Design review of the part built by this model. Coordinates are the model's own, in mm. A direction names the side the tool comes from. Round coordinates to 2 decimals unless told otherwise and drop trailing zeros. Loops run counter-clockwise (first coordinate to the right, second up) from the corner with the lowest first, then second, coordinate; pieces in that order, holes last. Notation, with made-up numbers: (-15.75, 81.5) - (0.25, 81.5) arc R6 cw to (0.25, 85.5) - close; hole circle Ø10 at (14, 35.25). An arc over 180 degrees is marked (long way). One line per question, with ' | ' between items. Start each with the question number.
from build123d import *

# Parameters (mm, degrees)
SKETCH1_W                = 53.5
SKETCH1_H                = 68.5
BOSS_EXTRUDE1_DEPTH      = 15
BOSS_EXTRUDE2_DEPTH      = 2.5
BOSS_EXTRUDE2_DEPTH_BACK = 15
SKETCH2_W                = 57.5
SKETCH2_H                = 72.5
SKETCH2_W_2              = 53.5
SKETCH2_H_2              = 68.5
SKETCH3_W                = 2.7
SKETCH3_H                = 68.5
CUT_EXTRUDE1_DEPTH       = 1.7
SKETCH4_R                = 1.3
CUT_EXTRUDE2_DEPTH       = 7
SKETCH5_W                = 15
SKETCH5_H                = 12
SKETCH5_R                = 2.5
SKETCH5_W_2              = 12
SKETCH5_H_2              = 15
BOSS_EXTRUDE3_DEPTH      = 3.5
FILLET1_R                = 5
FILLET2_R                = 3


with BuildPart() as part:
    # Sketch1 → Boss-Extrude1 (new body)
    with BuildSketch(Plane.XY):
        with Locations((26.75, 34.25)):
            Rectangle(SKETCH1_W, SKETCH1_H)
    extrude(amount=BOSS_EXTRUDE1_DEPTH)

    # Sketch2 → Boss-Extrude2 (add, two sides: drawn at the far end of the back side and taken through both)
    with BuildSketch(Plane.XY.offset(15).offset(-BOSS_EXTRUDE2_DEPTH_BACK)):
        with Locations((26.75, 34.25)):
            Rectangle(SKETCH2_W, SKETCH2_H)
        with Locations((26.75, 34.25)):
            Rectangle(SKETCH2_W_2, SKETCH2_H_2, mode=Mode.SUBTRACT)
    extrude(amount=BOSS_EXTRUDE2_DEPTH + BOSS_EXTRUDE2_DEPTH_BACK)

    # Sketch3 → Cut-Extrude1 (cut)
    with BuildSketch(Plane.XY.offset(15)):
        with Locations((1.85, 34.25)):
            Rectangle(SKETCH3_W, SKETCH3_H)
        with Locations((51.65, 34.25)):
            Rectangle(SKETCH3_W, SKETCH3_H)
    extrude(amount=-CUT_EXTRUDE1_DEPTH, mode=Mode.SUBTRACT)

    # Sketch4 → Cut-Extrude2 (cut)
    with BuildSketch(Plane.XY.offset(15)):
        with Locations((35.56, 12.7)):
            Circle(SKETCH4_R)
        with Locations((35.56, 60.96)):
            Circle(SKETCH4_R)
    extrude(amount=-CUT_EXTRUDE2_DEPTH, mode=Mode.SUBTRACT)

    # Sketch5 → Boss-Extrude3 (add)
    # profile 1 of 4: a face of its own
    with BuildSketch(Plane(origin=(0, 0, 0), x_dir=(-1, 0, 0), z_dir=(0, 0, -1))):
        with Locations((-26.75, -8)):
            Rectangle(SKETCH5_W, SKETCH5_H)
        with Locations((-26.75, -8)):
            Circle(SKETCH5_R, mode=Mode.SUBTRACT)
    # profile 2 of 4: a face of its own
    with BuildSketch(Plane(origin=(0, 0, 0), x_dir=(-1, 0, 0), z_dir=(0, 0, -1))):
        with Locations((8, 34.25)):
            Rectangle(SKETCH5_W_2, SKETCH5_H_2)
        with Locations((8, 34.25)):
            Circle(SKETCH5_R, mode=Mode.SUBTRACT)
    # profile 3 of 4: a face of its own
    with BuildSketch(Plane(origin=(0, 0, 0), x_dir=(-1, 0, 0), z_dir=(0, 0, -1))):
        with Locations((-61.5, 34.25)):
            Rectangle(SKETCH5_W_2, SKETCH5_H_2)
        with Locations((-61.5, 34.25)):
            Circle(SKETCH5_R, mode=Mode.SUBTRACT)
    # profile 4 of 4: a face of its own
    with BuildSketch(Plane(origin=(0, 0, 0), x_dir=(-1, 0, 0), z_dir=(0, 0, -1))):
        with Locations((-26.75, 76.5)):
            Rectangle(SKETCH5_W, SKETCH5_H)
        with Locations((-26.75, 76.5)):
            Circle(SKETCH5_R, mode=Mode.SUBTRACT)
    extrude(amount=-BOSS_EXTRUDE3_DEPTH)

    # Fillet1
    fillet1_edges = [part.edges().sort_by_distance(p)[0] for p in [
        (55.5, 41.75, 1.75),
        (55.5, 26.75, 1.75),
        (67.5, 26.75, 1.75),
        (67.5, 41.75, 1.75),
        (34.25, 70.5, 1.75),
        (34.25, 82.5, 1.75),
        (19.25, 82.5, 1.75),
        (19.25, 70.5, 1.75),
        (34.25, -14, 1.75),
        (34.25, -2, 1.75),
        (19.25, -2, 1.75),
        (19.25, -14, 1.75),
        (-2, 26.75, 1.75),
        (-2, 41.75, 1.75),
        (-14, 41.75, 1.75),
        (-14, 26.75, 1.75),
    ]]
    fillet(fillet1_edges, radius=FILLET1_R)

    # Fillet2
    fillet2_edges = [part.edges().sort_by_distance(p)[0] for p in [
        (55.5, 34.25, 3.5),
        (26.75, 70.5, 3.5),
        (26.75, -2, 3.5),
        (-2, 34.25, 3.5),
    ]]
    fillet(fillet2_edges, radius=FILLET2_R)


solid = part.part
1. Take a section at A-A, the plane x = 26.75. Give the boundary of the cut face in (y, z), then the cut area to 3 significant figures.
2. To check wall thickness, follow line 1 along Y through (x, z) = (26.75, 1.9); line 2 along Y through (x, z) = (36, 9.5); line 3 along Y through (x, z) = (32, 12.5). State the ranges of each line that lie inside material, in increasing order.
3. Clearance check with flat-ended pins moving along their axes: P1, Ø1, axis at x = 62, z = 1.5, coming from the +Y side; P2, Ø1, axis at y = 49.5, z = 12.5, coming from the -X side; P3, Ø6, axis at x = -0.5, z = 9.5, coming from the -Y side. State where each tip first meets the part, or that it passes through.
4. Take a section at C-C, the plane z = 9.75. Give the boundary of the cut face in (x, y), then the cut area to 3 significant figures.
5. Machinability: for faces 1 (the face through (56.37, 43.93, 2.57)), 2 (the face through (-8, 41.75, 2)), 3 (the face through (62, 26.75, 2)), 4 (the face through (29, 79, 3.5)), which of the approach directions +Z, -Z, +X, -X, +Y, -Y give a long, thin tool a straight path to every point of the face, cutting with its end or side? Answer none if there is none.
6. The part is to be moulded in two halves that separate along X. For faces 5 (the face through (2, 35, 13.3)), 6 (the face through (59.115, 35.001, 1.726)), 7 (the face through (17.07, 71.37, 2.57)), 8 (the face through (27, 82.5, 2)), say which applies: pulls with the +X half, pulls with the -X half, needs draft (parallel to the pull), parting line crosses it, or undercut.
7. Take a section at D-D, the plane y = 60.96. Give the boundary of the cut face in (x, z).
8. Take a section at B-B, the plane y = 34.25. Count the separate pieces of the cut face and the enclosed holes in it, then the cut area to 3 significant figures.
Answer list:
1) outline: (-14, 0) - (-10.5, 0) - (-10.5, 3.5) - (-14, 3.5) - close; (-5.5, 0) - (74, 0) - (74, 3.5) - (73.5, 3.5) arc R3 cw to (70.5, 6.5) - (70.5, 17.5) - (68.5, 17.5) - (68.5, 15) - (0, 15) - (0, 17.5) - (-2, 17.5) - (-2, 6.5) arc R3 cw to (-5, 3.5) - (-5.5, 3.5) - close; (79, 0) - (82.5, 0) - (82.5, 3.5) - (79, 3.5) - close | area: 1,150 mm²
2) line 1: y = -14 to -10.5, -5.5 to 74, 79 to 82.5 | line 2: y = -2 to 11.48, 13.92 to 59.74, 62.18 to 70.5 | line 3: y = -2 to 70.5
3) P1: stops at y = 41.75 | P2: stops at x = -2 | P3: stops at y = -2
4) outline: (-2, -2) - (55.5, -2) - (55.5, 70.5) - (-2, 70.5) - close; hole circle Ø2.6 at (35.56, 12.7); hole circle Ø2.6 at (35.56, 60.96) | area: 4,160 mm²
5) face 1: +Z, -Z, +X, +Y | face 2: +Z, -Z, -X, +Y | face 3: +Z, -Z, +X, -Y | face 4: +Z, +X, -X, +Y
6) face 5: undercut | face 6: undercut | face 7: pulls with the -X half | face 8: needs draft
7) outline: (-2, 0) - (55.5, 0) - (55.5, 17.5) - (53.5, 17.5) - (53.5, 15) - (53, 15) - (53, 13.3) - (50.3, 13.3) - (50.3, 15) - (36.86, 15) - (36.86, 8) - (34.26, 8) - (34.26, 15) - (3.2, 15) - (3.2, 13.3) - (0.5, 13.3) - (0.5, 15) - (0, 15) - (0, 17.5) - (-2, 17.5) - close
8) separate pieces: 3 | enclosed holes: 0 | area: 916 mm²
